Source: three-view drawing plus pictorial views. Frame: mm from the lowest corner of the part. Give positions to 0.01 mm unless a question says otherwise; leave off trailing zeros. Loops run counter-clockwise (first coordinate to the right, second up) from the corner with the lowest first, then second, coordinate; pieces in that order, holes last. Notation, with made-up numbers: (33.25, 77) - (55.25, 77) arc R21 cw to (55.25, 83) - close; hole circle Ø5 at (51.5, 42). An arc over 180 degrees is marked (long way). One line per item, written item: value.
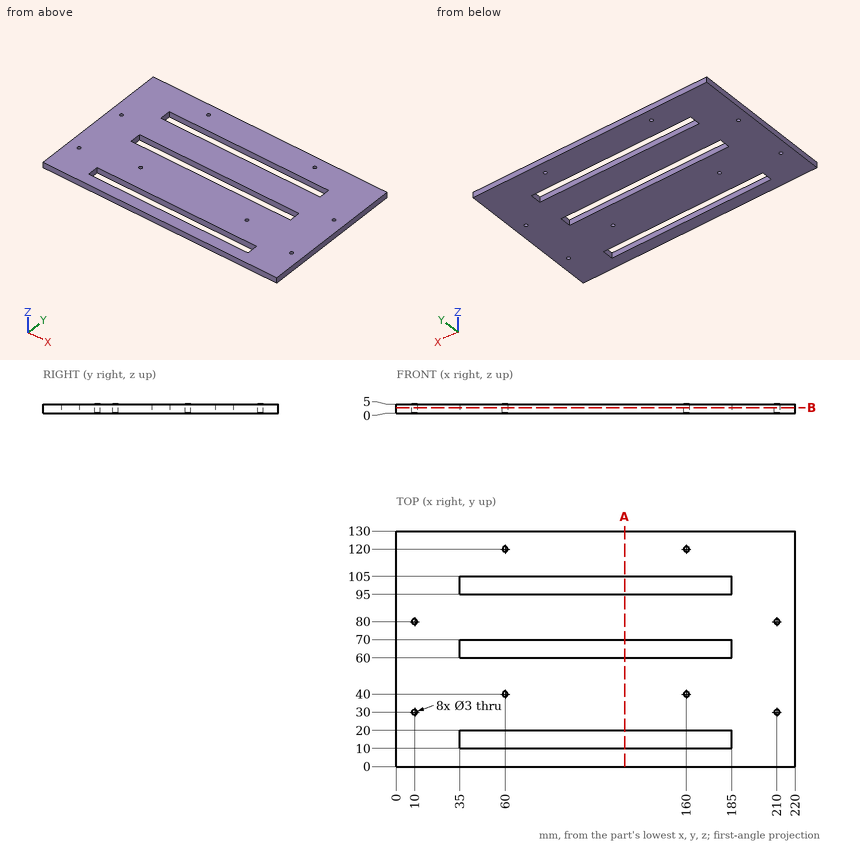
Item 1: Section A-A, the plane x = 126. Output: boundary loops of the cut face in (y, z).
Verdict:
outline: (0, 0) - (10, 0) - (10, 5) - (0, 5) - close; (20, 0) - (60, 0) - (60, 5) - (20, 5) - close; (70, 0) - (95, 0) - (95, 5) - (70, 5) - close; (105, 0) - (130, 0) - (130, 5) - (105, 5) - close
Item 2: Section B-B, the plane z = 2.95. Count the separate pieces of the cut face and the enclosed holes in it, and give its area (3 significant figures).
Verdict:
separate pieces: 1
enclosed holes: 11
area: 24,000 mm^2
Item 3: Material intervals for L1, parallel to Y at x = 97, z = 4; L2, parallel to X at y = 80, z = 2.05; L3, parallel to X at y = 40, z = 1.3, sorted ascending.
Verdict:
L1: y = 0 to 10, 20 to 60, 70 to 95, 105 to 130
L2: x = 0 to 8.5, 11.5 to 208.5, 211.5 to 220
L3: x = 0 to 58.5, 61.5 to 158.5, 161.5 to 220
Item 4: Pin query (flat end, axial travel): P1, Ø1.8, axis at x = 10, y = 80, coming from the -Z side. Return the tip coordinate at first contact, or that it passes through.
Verdict:
P1: passes through
